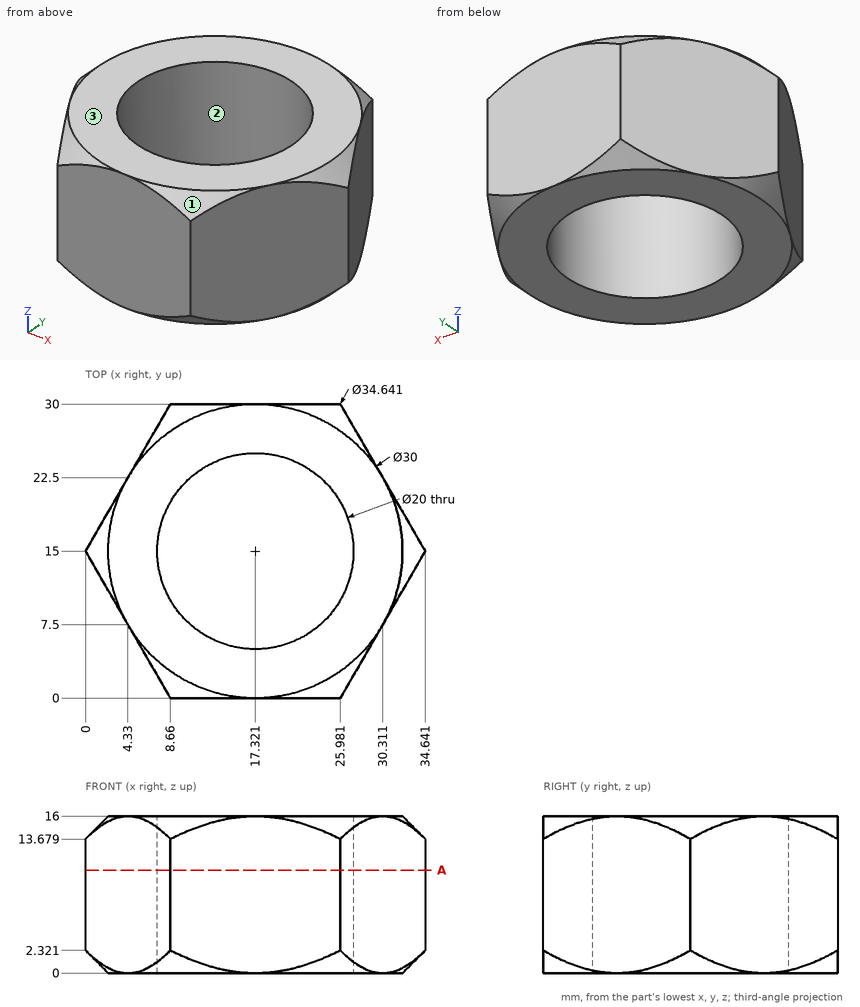
Could you check a few things on this drawing? It's one solid part, dimensions in mm from its lowest x, y, z. Coordinates: 2 decimals unless noted, no trailing zeros. Order: outer loops, then holes, each group sorted by start corner. A loop starts at its lowest first (then second) coordinate and runs counter-clockwise, first axis right, second up.
1) We'd pull the mould along X, two halves only. Please class the marked faces 1, 2 and 3: +X half, -X half, draft (parallel to the pull), parting line (faces both ways), or undercut.
2) Imagine slicing it at A-A on z = 10.5. List the corners of the cut face in (x, y) for me.
3) I need wall thicknesses on line 1 (Y direction, x = 22.5, z = 8) (1 decimal); line 2 (Y direction, x = 23, z = 9.25); line 3 (X direction, y = 17.25, z = 6) (1 decimal). Which ranges of each line are inside material? Lowest first, please.
4) Will these pins go through, and if not, where does the flat tip stop? pin 1 (3 mm diameter, centred on y = 22, z = 3, fed in from +X) (1 decimal); pin 2 (3 mm diameter, centred on x = 24, y = 9.5, fed in from +Z); pin 3 (5 mm diameter, centred on y = 3.5, z = 8.5, fed in from -X) (1 decimal); pin 4 (1.5 mm diameter, centred on y = 22, z = 13.5, fed in from +X).
Response values:
1. face 1: +X half
1. face 2: undercut
1. face 3: draft
2. outline: (0, 15) - (8.66, 0) - (25.98, 0) - (34.64, 15) - (25.98, 30) - (8.66, 30) - close; hole circle Ø20 at (17.32, 15)
3. line 1: y = 0 to 6.4, 23.6 to 30
3. line 2: y = 0 to 6.77, 23.23 to 30
3. line 3: x = 1.3 to 7.6, 27.1 to 33.3
4. pin 1: stops at x = 31.5
4. pin 2: stops at z = 16
4. pin 3: stops at x = 5.2
4. pin 4: stops at x = 31.03
